Here's how the part is built. I have some questions about the finished solid (model axes, mm). Face numbers are marked on the shaded views. A direction names the side the tool comes from. Give positions to 0.01 mm unless a question says otherwise; leave off trailing zeros. Loops run counter-clockwise (first coordinate to the right, second up) from the corner with the lowest first, then second, coordinate; pieces in that order, holes last. Notation, with made-up numbers: (49, 52.5) - (97, 52.5) arc R30 ccw to (97, 76.5) - close; hole circle Ø5 at (-31, 75). An arc over 180 degrees is marked (long way). Use one line per item in the form item = value.
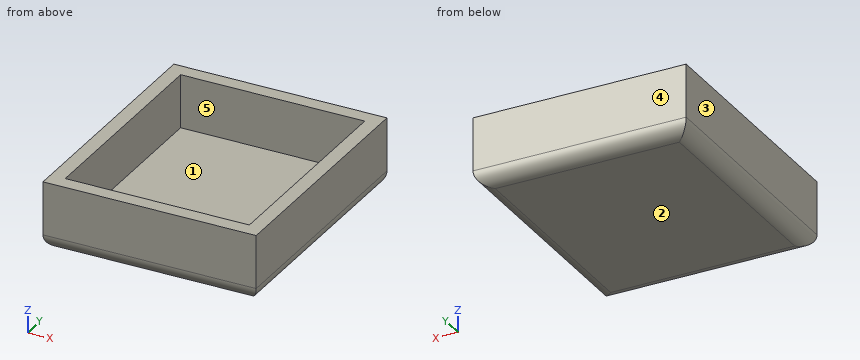
from build123d import *

# Parameters (mm, degrees)
SKETCH_1_W          = 44
SKETCH_1_H          = 51
EXTRUDE_2_DEPTH     = 14
SKETCH_2_W          = 38
SKETCH_2_H          = 45
CUT_EXTRUDE_1_DEPTH = 11
FILLET_1_R          = 3


with BuildPart() as part:
    # 草圖1 → 填料-伸長2 (new body)
    with BuildSketch(Plane.XY):
        with Locations((-37.776876722, -0.612244898)):
            Rectangle(SKETCH_1_W, SKETCH_1_H)
    extrude(amount=EXTRUDE_2_DEPTH)

    # 草圖2 → 除料-伸長1 (cut)
    with BuildSketch(Plane.XY.offset(14)):
        with Locations((-37.776876722, -0.612244898)):
            Rectangle(SKETCH_2_W, SKETCH_2_H)
    extrude(amount=-CUT_EXTRUDE_1_DEPTH, mode=Mode.SUBTRACT)

    # 圓角1
    fillet_1_edges = [part.edges().sort_by_distance(p)[0] for p in [
        (-37.776876722, 24.887755102, 0),
        (-15.776876722, -0.612244898, 0),
        (-37.776876722, -26.112244898, 0),
        (-59.776876722, -0.612244898, 0),
    ]]
    fillet(fillet_1_edges, radius=FILLET_1_R)


solid = part.part
(1) Thinking about a two-plate mould opening in X: for the marked faces 1, 2 and 3, which applies, pulls with the +X half, pulls with the -X half, needs draft (parallel to the pull), parting line crosses it, or undercut?
Geometry says:
face_1 = undercut
face_2 = needs draft
face_3 = pulls with the -X half
(2) If we section it at D-D (z = 1.25): List the corners of the cut face in (x, y) for me.
Geometry says:
outline = (-59.21, -25.55) - (-16.34, -25.55) - (-16.34, 24.32) - (-59.21, 24.32) - close
(3) If we section it at B-B (y = 16.5): List the corners of the cut face in (x, z) for me.
Geometry says:
outline = (-59.78, 3) arc R3 ccw to (-56.78, 0) - (-18.78, 0) arc R3 ccw to (-15.78, 3) - (-15.78, 14) - (-18.78, 14) - (-18.78, 3) - (-56.78, 3) - (-56.78, 14) - (-59.78, 14) - close
(4) If we section it at C-C (x = -23.5): List the corners of the cut face in (y, z) for me, plus the area to 3 significant figures.
Geometry says:
outline = (-26.11, 3) arc R3 ccw to (-23.11, 0) - (21.89, 0) arc R3 ccw to (24.89, 3) - (24.89, 14) - (21.89, 14) - (21.89, 3) - (-23.11, 3) - (-23.11, 14) - (-26.11, 14) - close
area = 215 mm²
(5) If I drill on probe 1 along X at (y, z) = (17.5, 13.25); probe 2 along Y at (x, z) = (-23, 8.5); probe 3 along Z at (x, y) = (-35, -2.5), over which ranges is the centre line in solid material (lowest first)?
Geometry says:
probe_1 = -59.78 to -56.78, -18.78 to -15.78
probe_2 = -26.11 to -23.11, 21.89 to 24.89
probe_3 = 0 to 3
(6) If we section it at A-A (z = 11.75): List the corners of the cut face in (x, y) for me.
Geometry says:
outline = (-59.78, -26.11) - (-15.78, -26.11) - (-15.78, 24.89) - (-59.78, 24.89) - close; hole (-56.78, -23.11) - (-18.78, -23.11) - (-18.78, 21.89) - (-56.78, 21.89) - close
(7) For P1, Ø4, axis at x = -52.5, y = -7, coming from the +Z side; P2, Ø6, axis at y = -6.5, z = 2.5, coming from the +X side, each with a flat end and sliding along its axis, tell me the tip position at first contact or that it passes through.
Geometry says:
P1 = 3
P2 = -15.78
(8) For the marked faces 4 and 5, which set-ups out of +Z, -Z, +X, -X, +Y, -Y let a thin tool reach every point of the face, with its end or its side?
Geometry says:
face_4 = +Z, -Z, +X, -X, +Y
face_5 = +Z
